Could you check a few things on this drawing? It's one solid part, dimensions in mm from its lowest x, y, z. A direction names the side the tool comes from. Give positions to 0.01 mm unless a question says otherwise; leave off trailing zeros. Order: outer loops, then holes, each group sorted by start corner. A loop starts at its lowest first (then second) coordinate and runs counter-clockwise, first axis right, second up. Notation, with made-up numbers: M 57,25.25 L 79,25.25 A12 ccw 79,38.25 Z; hole C 32.25,14 d9. An arc over 180 degrees is marked long. Use one line per item in the form item = value.
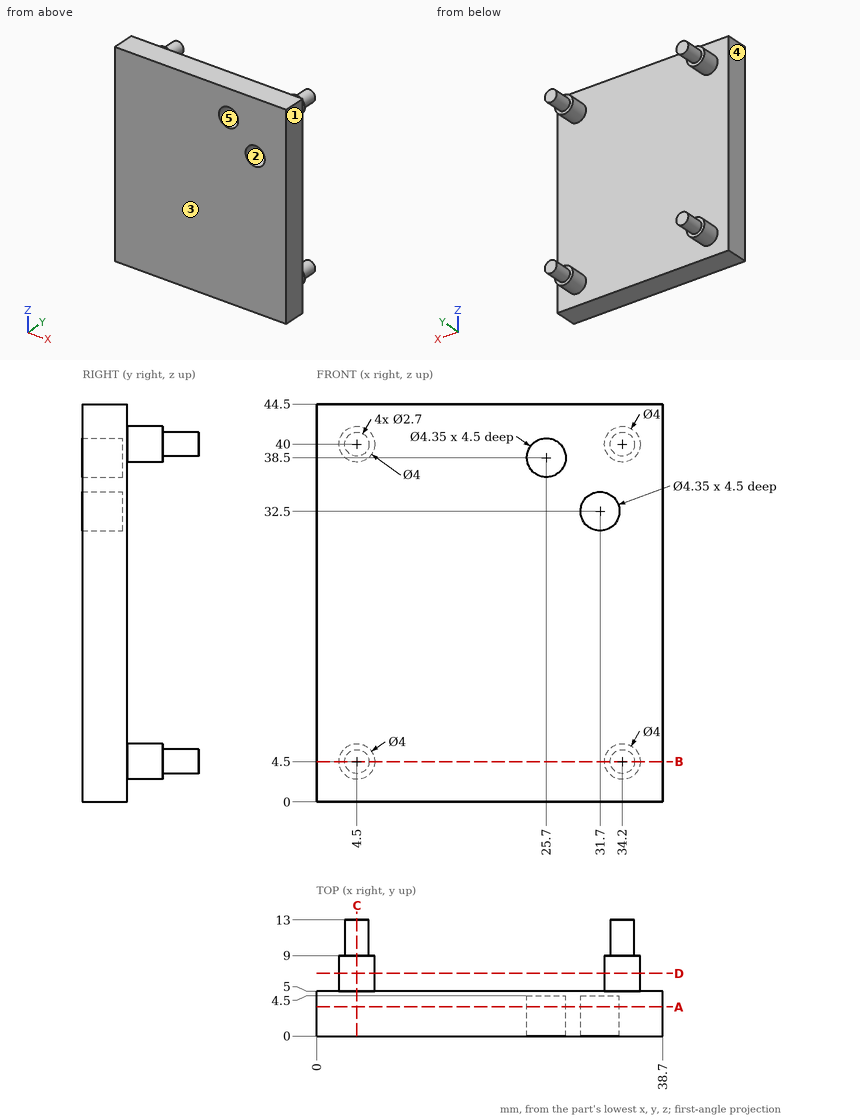
Q1. I'm going to push flat-ended pins straight in: pin 1 Ø4 at (x, z) = (31.7, 32.5) entering from -Y; pin 2 Ø3 at (x, z) = (25, 4.5) entering from +Y; pin 3 Ø2 at (y, z) = (9, 39.5) entering from -X. Where does each tip first touch, or does it pass through?
Found:
pin_1 = 4.5
pin_2 = 5
pin_3 = 2.5
Q2. I want a section at B-B on z = 4.5. Write out the boundary of the cut face in (x, y), then the cut area to 3 significant figures.
Found:
outline = M 0,0 L 38.7,0 L 38.7,5 L 36.2,5 L 36.2,9 L 35.55,9 L 35.55,13 L 32.85,13 L 32.85,9 L 32.2,9 L 32.2,5 L 6.5,5 L 6.5,9 L 5.85,9 L 5.85,13 L 3.15,13 L 3.15,9 L 2.5,9 L 2.5,5 L 0,5 Z
area = 247 mm²
Q3. I want a section at C-C on x = 4.5. Write out the boundary of the cut face in (y, z).
Found:
outline = M 0,0 L 5,0 L 5,2.5 L 9,2.5 L 9,3.15 L 13,3.15 L 13,5.85 L 9,5.85 L 9,6.5 L 5,6.5 L 5,38 L 9,38 L 9,38.65 L 13,38.65 L 13,41.35 L 9,41.35 L 9,42 L 5,42 L 5,44.5 L 0,44.5 Z
Q4. I want a section at A-A on y = 3.25. Write out the boundary of the cut face in (x, z) (3 decimals).
Found:
outline = M 0,0 L 38.7,0 L 38.7,44.5 L 0,44.5 Z; hole C 25.7,38.5 d4.35; hole C 31.7,32.5 d4.35
Q5. On a 3-axis mill with a long thin cutter (end or side, diameter ignored), from which of +Z, -Z, +X, -X, +Y, -Y can I reach the whole of each face in a straight line? I mean the marked faces 1 and 2. Say none if no direction works.
Found:
face_1 = +Z, -Z, +X, +Y, -Y
face_2 = -Y
Q6. Thinking about a two-plate mould opening in X: for the marked faces 3, 4 and 5, which applies, +X half, -X half, draft (parallel to the pull), parting line (faces both ways), or undercut?
Found:
face_3 = draft
face_4 = -X half
face_5 = undercut
Q7. I need wall thicknesses on L1, parallel to X at y = 3.3, z = 38.5 (3 decimals); L2, parallel to X at y = 1.75, z = 32.5 (3 decimals); L3, parallel to Y at x = 36.5, z = 26.5. Which ranges of each line are inside material? Lowest first, please.
Found:
L1 = 0 to 23.525, 27.875 to 38.7
L2 = 0 to 29.525, 33.875 to 38.7
L3 = 0 to 5
Q8. I want a section at D-D on y = 7. Write out the boundary of the cut face in (x, z), then the cut area to 3 significant figures.
Found:
outline = C 4.5,4.5 d4; C 4.5,40 d4; C 34.2,4.5 d4; C 34.2,40 d4
area = 50.3 mm²
